Input: part model. Units: mm. Frame: model coordinates. A direction names the side the tool comes from. Give positions to 0.01 mm unless a question says otherwise; leave off trailing zeros. Order: outer loops, then holes, each group sorted by start corner. A loop starts at its lowest first (then second) coordinate and runs counter-clockwise, first axis right, second up.
```python
from build123d import *

# Parameters (mm, degrees)
MAINBASESKETCH_W      = 7.9
MAINBASESKETCH_H      = 3.2
MAINBASEEXTRUDE_DEPTH = 7.9
MAINBASESHELL_T       = -1.2


with BuildPart() as part:
    # MainBaseSketch → MainBaseExtrude (new, symmetric)
    with BuildSketch(Plane.XY):
        with Locations((4.631967213, 1.6)):
            Rectangle(MAINBASESKETCH_W, MAINBASESKETCH_H)
    extrude(amount=MAINBASEEXTRUDE_DEPTH, both=True)

    # MainBaseShell
    mainbaseshell_openings = [part.faces().sort_by_distance(p)[0] for p in [
        (4.631967213, 0, 0),
    ]]
    offset(amount=MAINBASESHELL_T, openings=mainbaseshell_openings, kind=Kind.INTERSECTION)


solid = part.part
```
1) Pull-direction query (Z, two-part tool) for faces 1 (the face through (5, 2, -7.9)), 2 (the face through (1.882, 1, 0)), 3 (the face through (5, 3.2, 0)); classes: pulls with the +Z half, pulls with the -Z half, needs draft (parallel to the pull), parting line crosses it, or undercut.
2) Cut plane A-A (z = -0.5). Return the cut outline in (x, y).
3) Cut plane C-C (x = 5.5). Return the cut outline in (y, z), then the cut area to 3 significant figures.
4) Reachability of faces 4 (the face through (5, 1, -6.7)), 5 (the face through (0.682, 2, 0)) from +Z, -Z, +X, -X, +Y, -Y: full face, straight path, thin tool, end or side. Return the list, or none.
5) Line query: probe 1 along Z at (x, y) = (7, 1.5); probe 2 along X at (y, z) = (1.2, -6.5); probe 3 along Y at (x, z) = (6, 1.5). Output: solid intervals per line, ascending.
6) Cut plane B-B (y = 1). Return the cut outline in (x, z).
Geometry says:
1. face 1: pulls with the -Z half
1. face 2: undercut
1. face 3: needs draft
2. outline: (0.68, 0) - (1.88, 0) - (1.88, 2) - (7.38, 2) - (7.38, 0) - (8.58, 0) - (8.58, 3.2) - (0.68, 3.2) - close
3. outline: (0, -7.9) - (3.2, -7.9) - (3.2, 7.9) - (0, 7.9) - (0, 6.7) - (2, 6.7) - (2, -6.7) - (0, -6.7) - close
3. area: 23.8 mm2
4. face 4: -Y
4. face 5: +Z, -Z, -X, +Y, -Y
5. probe 1: z = -7.9 to -6.7, 6.7 to 7.9
5. probe 2: x = 0.68 to 1.88, 7.38 to 8.58
5. probe 3: y = 2 to 3.2
6. outline: (0.68, -7.9) - (8.58, -7.9) - (8.58, 7.9) - (0.68, 7.9) - close; hole (1.88, -6.7) - (7.38, -6.7) - (7.38, 6.7) - (1.88, 6.7) - close
